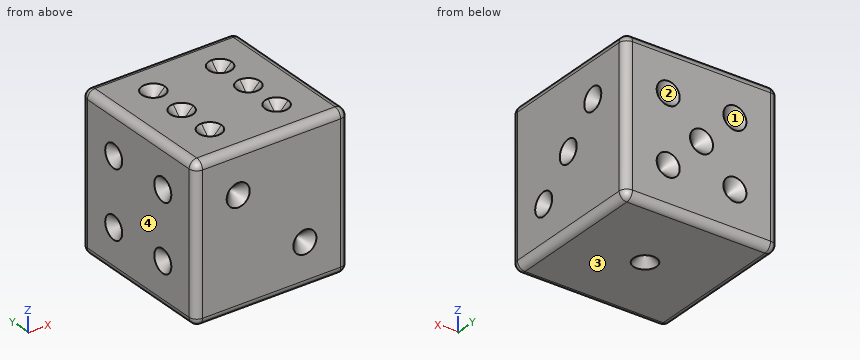
```python
from build123d import *

# Parameters (mm, degrees)
F0_W      = 20
F0_H      = 20
F1_DEPTH  = 20
F2_R      = 1.5
F3_DEPTH  = 1.5
F4_R      = 1
F5_R      = 1.5
F6_DEPTH  = 1.5
F7_R      = 1.5
F8_DEPTH  = 1.5
F9_SIZE   = 1.49999
F10_SIZE  = 1.49999
F11_SIZE  = 1.49999
F12_R     = 1.5
F13_DEPTH = 1.5
F14_SIZE  = 1.49999
F15_R     = 1.5
F16_DEPTH = 1.5
F17_SIZE  = 1.49999
F19_DEPTH = 1.5
F20_SIZE  = 1.49999


# Not quite as in the source:
# - a fillet or chamfer is up to 0.001 mm smaller than in the source, because OpenCascade refuses the exact size


with BuildPart() as f1:
    # F0 (on Top) → F1 (new body)
    with BuildSketch(Plane.XY):
        with Locations((10, 10)):
            Rectangle(F0_W, F0_H)
    extrude(amount=F1_DEPTH)

    # F2 (on face) → F3 (cut)
    with BuildSketch(Plane.XZ):
        with Locations((5.6568542495, 14.3431457505)):
            Circle(F2_R)
        with Locations((14.3431457505, 5.6568542495)):
            Circle(F2_R)
    extrude(amount=-F3_DEPTH, mode=Mode.SUBTRACT)

    # F4
    f4_edges = [f1.edges().sort_by_distance(p)[0] for p in [
        (10, 0, 20),
        (20, 0, 10),
        (10, 0, 0),
        (0, 0, 10),
        (20, 10, 0),
        (10, 20, 0),
        (0, 10, 0),
        (20, 20, 10),
        (20, 10, 20),
        (10, 20, 20),
        (0, 10, 20),
        (0, 20, 10),
    ]]
    fillet(f4_edges, radius=F4_R)

    # F5 (on face) → F6 (cut)
    with BuildSketch(Plane.XY):
        with Locations((10, 10)):
            Circle(F5_R)
    extrude(amount=F6_DEPTH, mode=Mode.SUBTRACT)

    # F7 (on Right) → F8 (cut)
    with BuildSketch(Plane.YZ):
        with Locations((5.6568542495, 14.3431457505)):
            Circle(F7_R)
        with Locations((14.3431457505, 14.3431457505)):
            Circle(F7_R)
        with Locations((14.3431457505, 5.6568542495)):
            Circle(F7_R)
        with Locations((5.6568542495, 5.6568542495)):
            Circle(F7_R)
    extrude(amount=F8_DEPTH, mode=Mode.SUBTRACT)

    # F9 (size 1.5 in the source; OpenCascade refuses exactly that, so slightly less here)
    f9_edges = [f1.edges().sort_by_distance(p)[0] for p in [
        (4.156854, 1.5, 14.343146),
        (12.843146, 1.5, 5.656854),
    ]]
    chamfer(f9_edges, length=F9_SIZE)

    # F10 (size 1.5 in the source; OpenCascade refuses exactly that, so slightly less here)
    f10_edges = [f1.edges().sort_by_distance(p)[0] for p in [
        (1.5, 12.843146, 14.343146),
        (1.5, 4.156854, 14.343146),
        (1.5, 4.156854, 5.656854),
        (1.5, 12.843146, 5.656854),
    ]]
    chamfer(f10_edges, length=F10_SIZE)

    # F11 (size 1.5 in the source; OpenCascade refuses exactly that, so slightly less here)
    f11_edges = [f1.edges().sort_by_distance(p)[0] for p in [
        (8.5, 10, 1.5),
    ]]
    chamfer(f11_edges, length=F11_SIZE)

    # F12 (on face) → F13 (cut)
    with BuildSketch(Plane.YZ.offset(20)):
        with Locations((5.6568542495, 5.6568542495)):
            Circle(F12_R)
        with Locations((10, 10)):
            Circle(F12_R)
        with Locations((14.3431457505, 14.3431457505)):
            Circle(F12_R)
    extrude(amount=-F13_DEPTH, mode=Mode.SUBTRACT)

    # F14 (size 1.5 in the source; OpenCascade refuses exactly that, so slightly less here)
    f14_edges = [f1.edges().sort_by_distance(p)[0] for p in [
        (18.5, 8.5, 10),
        (18.5, 12.843146, 14.343146),
        (18.5, 4.156854, 5.656854),
    ]]
    chamfer(f14_edges, length=F14_SIZE)

    # F15 (on face) → F16 (cut)
    with BuildSketch(Plane(origin=(0, 20, 0), x_dir=(-1, 0, 0), z_dir=(0, 1, 0))):
        with Locations((-14.3431457505, 14.3431457505)):
            Circle(F15_R)
        with Locations((-5.6568542495, 5.6568542495)):
            Circle(F15_R)
        with Locations((-14.3431457505, 5.6568542495)):
            Circle(F15_R)
        with Locations((-5.6568542495, 14.3431457505)):
            Circle(F15_R)
        with Locations((-10, 10)):
            Circle(F15_R)
    extrude(amount=-F16_DEPTH, mode=Mode.SUBTRACT)

    # F17 (size 1.5 in the source; OpenCascade refuses exactly that, so slightly less here)
    f17_edges = [f1.edges().sort_by_distance(p)[0] for p in [
        (15.843146, 18.5, 14.343146),
        (7.156854, 18.5, 14.343146),
        (11.5, 18.5, 10),
        (15.843146, 18.5, 5.656854),
        (7.156854, 18.5, 5.656854),
    ]]
    chamfer(f17_edges, length=F17_SIZE)

    # F18 (on face) → F19 (cut)
    with BuildSketch(Plane.XY.offset(20)):
        with BuildLine():
            ThreePointArc((7.1568542495, 15), (4.5961940777, 16.0606601718), (5.6568542495, 13.5))
            ThreePointArc((5.6568542495, 13.5), (6.7175144213, 13.9393398282), (7.1568542495, 15))
        make_face()
        with BuildLine():
            ThreePointArc((5.6568542495, 11.5), (4.1568542495, 10), (5.6568542495, 8.5))
            Line((5.6568542495, 8.5), (5.6568542495, 10))
            Line((5.6568542495, 10), (5.6568542495, 11.5))
        make_face()
        with BuildLine():
            Line((5.6568542495, 10), (5.6568542495, 8.5))
            ThreePointArc((5.6568542495, 8.5), (6.7175144213, 8.9393398282), (7.1568542495, 10))
            ThreePointArc((7.1568542495, 10), (6.7175144213, 11.0606601718), (5.6568542495, 11.5))
            Line((5.6568542495, 11.5), (5.6568542495, 10))
        make_face()
        with BuildLine():
            ThreePointArc((5.6568542495, 6.5), (4.1568542495, 5), (5.6568542495, 3.5))
            Line((5.6568542495, 3.5), (5.6568542495, 5))
            Line((5.6568542495, 5), (5.6568542495, 6.5))
        make_face()
        with BuildLine():
            Line((5.6568542495, 5), (5.6568542495, 3.5))
            ThreePointArc((5.6568542495, 3.5), (6.7175144213, 3.9393398282), (7.1568542495, 5))
            ThreePointArc((7.1568542495, 5), (6.7175144213, 6.0606601718), (5.6568542495, 6.5))
            Line((5.6568542495, 6.5), (5.6568542495, 5))
        make_face()
        with BuildLine():
            ThreePointArc((14.3431457505, 16.5), (12.8431457505, 15), (14.3431457505, 13.5))
            Line((14.3431457505, 13.5), (14.3431457505, 15))
            Line((14.3431457505, 15), (14.3431457505, 16.5))
        make_face()
        with BuildLine():
            Line((14.3431457505, 15), (14.3431457505, 13.5))
            ThreePointArc((14.3431457505, 13.5), (15.4038059223, 13.9393398282), (15.8431457505, 15))
            ThreePointArc((15.8431457505, 15), (15.4038059223, 16.0606601718), (14.3431457505, 16.5))
            Line((14.3431457505, 16.5), (14.3431457505, 15))
        make_face()
        with BuildLine():
            ThreePointArc((14.3431457505, 11.5), (12.8431457505, 10), (14.3431457505, 8.5))
            Line((14.3431457505, 8.5), (14.3431457505, 10))
            Line((14.3431457505, 10), (14.3431457505, 11.5))
        make_face()
        with BuildLine():
            Line((14.3431457505, 10), (14.3431457505, 8.5))
            ThreePointArc((14.3431457505, 8.5), (15.4038059223, 8.9393398282), (15.8431457505, 10))
            ThreePointArc((15.8431457505, 10), (15.4038059223, 11.0606601718), (14.3431457505, 11.5))
            Line((14.3431457505, 11.5), (14.3431457505, 10))
        make_face()
        with BuildLine():
            ThreePointArc((14.3431457505, 6.5), (12.8431457505, 5), (14.3431457505, 3.5))
            Line((14.3431457505, 3.5), (14.3431457505, 5))
            Line((14.3431457505, 5), (14.3431457505, 6.5))
        make_face()
        with BuildLine():
            Line((14.3431457505, 5), (14.3431457505, 3.5))
            ThreePointArc((14.3431457505, 3.5), (15.4038059223, 3.9393398282), (15.8431457505, 5))
            ThreePointArc((15.8431457505, 5), (15.4038059223, 6.0606601718), (14.3431457505, 6.5))
            Line((14.3431457505, 6.5), (14.3431457505, 5))
        make_face()
    extrude(amount=-F19_DEPTH, mode=Mode.SUBTRACT)

    # F20 (size 1.5 in the source; OpenCascade refuses exactly that, so slightly less here)
    f20_edges = [f1.edges().sort_by_distance(p)[0] for p in [
        (5.656854, 6.5, 18.5),
        (5.656854, 11.5, 18.5),
        (5.656854, 16.5, 18.5),
        (14.343146, 16.5, 18.5),
        (14.343146, 6.5, 18.5),
        (14.343146, 11.5, 18.5),
    ]]
    chamfer(f20_edges, length=F20_SIZE)


solid = f1.part
```
Could you check a few things on this model? Use its own coordinates, in mm. Face numbers are marked on the shaded views. Round coordinates to 2 decimals unless told otherwise and drop trailing zeros. Write item = value, one per line.
1. Will these pins go through, and if not, where does the flat tip stop? P1, Ø2.5, axis at x = 14.34, z = 5.66, coming from the -Y side; P2, Ø2.5, axis at y = 10, z = 10, coming from the +X side.
Results below:
P1 = 0.25
P2 = 19.75
2. I need wall thicknesses on probe 1 along Y at (x, z) = (15, 15); probe 2 along X at (y, z) = (2.25, 19.25); probe 3 along X at (y, z) = (9.5, 9.75). Which ranges of each line are inside material? Lowest first, please.
Results below:
probe_1 = 0 to 19.43
probe_2 = 0.03 to 19.97
probe_3 = 0 to 19.06
3. Thinking about a two-plate mould opening in X: for the marked faces 1, 2, 3 and 4, which applies, +X half, -X half, draft (parallel to the pull), parting line (faces both ways), or undercut?
Results below:
face_1 = undercut
face_2 = undercut
face_3 = draft
face_4 = -X half
